Verification items for the finished model (mm, model axes). A direction names the side the tool comes from. Round coordinates to 2 decimals unless told otherwise and drop trailing zeros. Order: outer loops, then holes, each group sorted by start corner. A loop starts at its lowest first (then second) coordinate and runs counter-clockwise, first axis right, second up. Notation, with made-up numbers: M 29.25,89 L 55.25,89 A29 cw 55.25,124 Z; hole C 2,49 d8. An arc over 180 degrees is marked long. Use one line per item in the form item = value. Start each with the question number.
Item 1: Tool access check on faces 4 (the cylindrical face through (189.04, 180.68, 1.48)), 5 (the flat face through (185, 187.339, 1)). Record the directions out of +Z, -Z, +X, -X, +Y, -Y that give a thin tool (end or side, any length) a straight path to the whole face; none if there is none.
Item 2: Cross-section at B-B on y = 170. Enter the section's corners in (x, z).
Item 3: Cross-section at C-C on x = 211.5. Enter the section's corners in (y, z), then the cut area to 3 significant figures.
Item 4: Go/stop test with flat-tipped pins: pin 1 Ø1 at (y, z) = (188.5, 1) entering from -X; pin 2 Ø1.4 at (x, z) = (195.5, 2) entering from +Y; pin 3 Ø2.5 at (x, y) = (172.8, 180.53) entering from -Z; pin 4 Ø0.7 at (y, z) = (188.5, 1) entering from +X. Record where each tip stops, or that it passes through.
Item 5: Release check for a two-part mould opening along X. For faces 1 (the flat face through (191, 180, 0)), 2 (the flat face through (186.356, 188.5, 1.5)), 3 (the cylindrical face through (174.188, 179.952, 1.479)) record: +X half, -X half, draft (parallel to the pull), parting line (faces both ways), or undercut.
Item 6: Cross-section at A-A on z = 2.3. Enter the section's corners in (x, y).
Item 7: Thickness scan on probe 1 along X at (y, z) = (181.75, 1.75); probe 2 along X at (y, z) = (180.25, 1.05); probe 3 along X at (y, z) = (180, 0.7). Record the ranges inside material, lowest first. Write a range as [from, to].
Item 8: Cross-section at D-D on y = 177.5. Enter the section's corners in (x, z), then the cut area to 3 significant figures.
from build123d import *

# Parameters (mm, degrees)
MODEL_R                 = 1.5
SALIENTE_EXTRUIR1_DEPTH = 3


with BuildPart() as part:
    # Model → Saliente-Extruir1 (new body)
    with BuildSketch(Plane.XY):
        with BuildLine():
            Line((191.396871733, 188.964281637), (194.105949351, 188.964281637))
            Line((194.105949351, 188.964281637), (194.105949351, 188.089281637))
            ThreePointArc((194.105949351, 188.089281637), (194.325619265, 187.558951551), (194.855949351, 187.339281637))
            Line((194.855949351, 187.339281637), (196.605949351, 187.339281637))
            ThreePointArc((196.605949351, 187.339281637), (197.136279437, 187.558951551), (197.355949351, 188.089281637))
            Line((197.355949351, 188.089281637), (197.355949351, 188.964281637))
            Line((197.355949351, 188.964281637), (215.17808095, 188.964281637))
            ThreePointArc((215.17808095, 188.964281637), (208.476468276, 173.498317967), (193.480949351, 165.80143179))
            ThreePointArc((193.480949351, 165.80143179), (174.362087289, 171.27143453), (165.283817753, 188.964281637))
            Line((165.283817753, 188.964281637), (183.105949351, 188.964281637))
            Line((183.105949351, 188.964281637), (183.105949351, 188.089281637))
            ThreePointArc((183.105949351, 188.089281637), (183.325619265, 187.558951551), (183.855949351, 187.339281637))
            Line((183.855949351, 187.339281637), (185.605949351, 187.339281637))
            ThreePointArc((185.605949351, 187.339281637), (186.136279437, 187.558951551), (186.355949351, 188.089281637))
            Line((186.355949351, 188.089281637), (186.355949351, 188.964281637))
            Line((186.355949351, 188.964281637), (189.06502697, 188.964281637))
            ThreePointArc((189.06502697, 188.964281637), (190.230949351, 188.589281637), (191.396871733, 188.964281637))
        make_face()
        with Locations((172.802524293, 180.526975738)):
            Circle(MODEL_R, mode=Mode.SUBTRACT)
        with Locations((190.230949351, 170.464669839)):
            Circle(MODEL_R, mode=Mode.SUBTRACT)
        with Locations((207.659374409, 180.526975738)):
            Circle(MODEL_R, mode=Mode.SUBTRACT)
        with Locations((190.230949351, 181.589281637)):
            Circle(MODEL_R, mode=Mode.SUBTRACT)
    extrude(amount=SALIENTE_EXTRUIR1_DEPTH)


solid = part.part
Output values:
q1.face_4 = +Z, -Z
q1.face_5 = +Z, -Z, +Y
q2.outline = M 176.05,0 L 188.8,0 L 188.8,3 L 176.05,3 Z; M 191.66,0 L 204.41,0 L 204.41,3 L 191.66,3 Z
q3.outline = M 177.45,0 L 188.96,0 L 188.96,3 L 177.45,3 Z
q3.area = 34.5 mm2
q4.pin_1 = 165.28
q4.pin_2 = 187.34
q4.pin_3 = through
q4.pin_4 = 215.17
q5.face_1 = draft
q5.face_2 = undercut
q5.face_3 = undercut
q6.outline = M 165.28,188.96 A25 ccw 215.18,188.96 L 197.36,188.96 L 197.36,188.09 A0.75 cw 196.61,187.34 L 194.86,187.34 A0.75 cw 194.11,188.09 L 194.11,188.96 L 191.4,188.96 A2 cw 189.07,188.96 L 186.36,188.96 L 186.36,188.09 A0.75 cw 185.61,187.34 L 183.86,187.34 A0.75 cw 183.11,188.09 L 183.11,188.96 Z; hole C 172.8,180.53 d3; hole C 190.23,170.46 d3; hole C 190.23,181.59 d3; hole C 207.66,180.53 d3
q7.probe_1 = [166.85, 171.93], [173.67, 188.74], [191.72, 206.79], [208.53, 213.62]
q7.probe_2 = [167.47, 171.33], [174.28, 189.56], [190.91, 206.19], [209.13, 212.99]
q7.probe_3 = [167.58, 171.4], [174.21, 206.25], [209.06, 212.88]
q8.outline = M 168.93,0 L 211.53,0 L 211.53,3 L 168.93,3 Z
q8.area = 128 mm2
